The model under review builds one solid part; all positions refer to its coordinate system, in mm. A direction names the side the tool comes from. Round coordinates to 2 decimals unless told otherwise and drop trailing zeros. Loops run counter-clockwise (first coordinate to the right, second up) from the corner with the lowest first, then second, coordinate; pieces in that order, holes last. Notation, with made-up numbers: (32.5, -31.75) -> (59.5, -31.75) arc R21 ccw to (59.5, -1.75) -> close; hole circle Ø3 at (-9, -38). An arc over 180 degrees is marked (long way). Write each question's results on one line, items separated by ' | '. Start each with the question number.
Item 1: We need section A-A (z = -3). Give the boundary of the cut face in (x, y).
Item 2: For L1, parallel to Y at x = 0.1, z = -3.75; L2, parallel to Y at x = 0.1, z = 0.75, list the stretches that pass through material, from the lowest coordinate up. Write a range as from..to.
Item 3: Clearance check with flat-ended pins moving along their axes: pin 1 Ø1 at (y, z) = (-1.5, -2) entering from -X; pin 2 Ø1.5 at (x, y) = (1, 2) entering from +Z; pin 3 Ø2 at (y, z) = (-1.5, -6.5) entering from -X. State where each tip first meets the part, or that it passes through.
Item 4: Tool access review of faces 1 (the flat face through (0, 0, -10)), 2 (the flat face through (-1, 0, 1)), 3 (the cylindrical face through (1.43, -0.45, -4.86)): name each direction out of +Z, -Z, +X, -X, +Y, -Y from which nothing blocks a thin tool from reaching the whole face with its end or side.
Item 5: Mouldability with a two-part tool opening along X and no side actions: class faces 4 (the flat face through (-2, 0, 0)), 5 (the flat face through (1, 0, 1)), 6 (the cylindrical face through (1.27, 2.44, 0.15)) as pulls with the +X half, pulls with the -X half, needs draft (parallel to the pull), parting line crosses it, or undercut.
from build123d import *

# Parameters (mm, degrees)
CHAMFER1_SIZE      = 0.25
CUT_EXTRUDE1_START = -1.4000001
CUT_EXTRUDE1_DEPTH = 1.4000001
FILLET1_R          = 0.1


with BuildPart() as part:
    # Sketch1 → Revolve1 (revolve)
    with BuildSketch(Plane(origin=(0, 0, 0), x_dir=(0, 0, -1), z_dir=(1, 0, 0)), mode=Mode.PRIVATE) as revolve1_sk:
        with BuildLine():
            Line((10, 0), (10, 1.5))
            Line((10, 1.5), (0, 1.5))
            Line((0, 1.5), (0, 2.75))
            Line((0, 2.75), (-0.3, 2.75))
            ThreePointArc((-0.3, 2.75), (-1.39323202, 2.363223225), (-2, 1.375))
            Line((-2, 1.375), (-2, 0))
            Line((-2, 0), (10, 0))
        make_face()
    revolve(revolve1_sk.sketch.rotate(Axis((0, 0, 30.809969789), (0, 0, -1)), 90), axis=Axis((0, 0, 30.809969789), (0, 0, -1)))

    # Chamfer1
    chamfer1_edges = [part.edges().sort_by_distance(p)[0] for p in [
        (-1.5, 0, -10),
    ]]
    chamfer(chamfer1_edges, length=CHAMFER1_SIZE)

    # Sketch2 → Cut-Revolve1 (revolve, cut)
    with BuildSketch(Plane(origin=(0, 0, 0), x_dir=(0, 0, -1), z_dir=(1, 0, 0)), mode=Mode.PRIVATE) as cut_revolve1_sk:
        Polygon((-2, 0), (-2, 1), (-0.6, 1), (-0.022649731, 0), align=None)
    revolve(cut_revolve1_sk.sketch.rotate(Axis((0, 0, 2.452500839), (0, 0, -1)), 90), axis=Axis((0, 0, 2.452500839), (0, 0, -1)), mode=Mode.SUBTRACT)

    # Cut-Extrude1: read off the stored shape, not the designer's step
    # Cut-Extrude1 outline → Cut-Extrude1 (cut)
    with BuildSketch(Plane.XY.offset(2).offset(CUT_EXTRUDE1_START)):
        with BuildLine():
            Line((1, 0), (1, 0.577350269))
            Line((1, 0.577350269), (0.500019222, 0.866014306))
            ThreePointArc((0.500019222, 0.866014306), (0.866030953, 0.499990389), (1, 0))
        make_face()
        with BuildLine():
            ThreePointArc((-0.500019222, 0.866014306), (0, 1), (0.500019222, 0.866014306))
            Line((0.500019222, 0.866014306), (0, 1.154700538))
            Line((0, 1.154700538), (-0.500019222, 0.866014306))
        make_face()
        with BuildLine():
            Line((1, -0.577350269), (1, 0))
            ThreePointArc((1, 0), (0.866030953, -0.499990389), (0.500019222, -0.866014306))
            Line((0.500019222, -0.866014306), (1, -0.577350269))
        make_face()
        with BuildLine():
            ThreePointArc((-1, 0), (-0.866030953, 0.499990389), (-0.500019222, 0.866014306))
            Line((-0.500019222, 0.866014306), (-1, 0.577350269))
            Line((-1, 0.577350269), (-1, 0))
        make_face()
        with BuildLine():
            Line((0, -1.154700538), (0.500019222, -0.866014306))
            ThreePointArc((0.500019222, -0.866014306), (0, -1), (-0.500019222, -0.866014306))
            Line((-0.500019222, -0.866014306), (0, -1.154700538))
        make_face()
        with BuildLine():
            ThreePointArc((-0.500019222, -0.866014306), (-0.866030953, -0.499990389), (-1, 0))
            Line((-1, 0), (-1, -0.577350269))
            Line((-1, -0.577350269), (-0.500019222, -0.866014306))
        make_face()
    extrude(amount=CUT_EXTRUDE1_DEPTH, mode=Mode.SUBTRACT)

    # Cut-Extrude1 2 outline → Cut-Extrude1 2 (revolve)
    with BuildSketch(Plane.XZ):
        Polygon((1.154700598, 0.689316432), (0.999999957, 0.599999975), (1.154700538, 0.5999999), align=None)
    revolve(axis=Axis((0, 0, 0), (0, 0, 1)))

    # Fillet1
    fillet1_edges = [part.edges().sort_by_distance(p)[0] for p in [
        (-1.5, 0, 0),
    ]]
    fillet(fillet1_edges, radius=FILLET1_R)


solid = part.part
Here are the results:
1) outline: circle Ø3 at (0, 0)
2) L1: y = -1.5..1.5 | L2: y = -2.69..-1.1, 1.1..2.69
3) pin 1: stops at x = -1.12 | pin 2: stops at z = 1.97 | pin 3: stops at x = -1.41
4) face 1: -Z, +X, -X, +Y, -Y | face 2: +Z | face 3: -Z
5) face 4: needs draft | face 5: undercut | face 6: parting line crosses it
